Can you work these out from the model? Positions are in its coordinate system, mm. A direction names the side the tool comes from. Round coordinates to 2 decimals unless told otherwise and drop trailing zeros. Write each loop counter-clockwise with the first axis right and the second up, starting at its lowest first coordinate (ties: lowest second). Pieces come first, ordered by that corner, then holes. Notation, with made-up numbers: (-18.5, 49.25) -> (20.5, 49.25) arc R30 ccw to (20.5, 86.25) -> close; hole circle Ø5 at (7.5, 79.25). An arc over 180 degrees is marked (long way). Write item = value, one per line. Start each with the question number.
1) For faces 1 (the face through (3.4, 22.58, -11.66)), 2 (the face through (-4, 26, -23)), 3 (the face through (-12.057, 33.505, -11.339)), which set-ups out of +Z, -Z, +X, -X, +Y, -Y let a thin tool reach every point of the face, with its end or its side?
2) I'm going to push flat-ended pins straight in: pin 1 (9 mm diameter, centred on x = -2.5, z = -9.5, fed in from -Y); pin 2 (5.5 mm diameter, centred on x = -1.5, z = -10.5, fed in from +Y). Where does each tip first touch, or does it pass through?
3) Thinking about a two-plate mould opening in X: for faces 4 (the face through (8.84, 26.73, -11.34)), 5 (the face through (-19.5, 33.47, -11.66)), 6 (the face through (12.612, 26, -11)), 7 (the face through (8, 34.075, -11)), which applies, +X half, -X half, draft (parallel to the pull), parting line (faces both ways), or undercut?
4) Imagine slicing it at A-A, the plane x = 7. Please give me the cut outline in (y, z), then the cut area to 3 significant figures.
5) Imagine slicing it at B-B, the plane y = 21.75. Please give me the cut outline in (x, z).
6) If I drill on line 1 (Y direction, x = 7.5, z = -10.25); line 2 (X direction, y = 31.5, z = -15.75); line 3 (X direction, y = 25.5, z = -16), over which ranges is the centre line in solid material (lowest first)?
7) Imagine slicing it at D-D, the plane x = -7. Please give me the cut outline in (y, z), then the cut area to 3 significant figures.
8) Imagine slicing it at C-C, the plane z = -3.5. Please give me the cut outline in (x, y).
from build123d import *

# Parameters (mm, degrees)
SKETCH_1_W          = 32.677388302
SKETCH_1_H          = 15.432977872
EXTRUDE_1_DEPTH     = 23
SKETCH_2_R          = 1.25
SKETCH_2_W          = 15.458117654
SKETCH_2_H          = 9.017063249
CUT_EXTRUDE_1_DEPTH = 24
FILLET_1_R          = 2
FILLET_2_R          = 2


with BuildPart() as part:
    # 草图1 → 凸台-拉伸1 (new body)
    with BuildSketch(Plane.XY):
        with Locations((-3.726697353, 26.358574689)):
            Rectangle(SKETCH_1_W, SKETCH_1_H)
    extrude(amount=-EXTRUDE_1_DEPTH)

    # 草图2 → 切除-拉伸1 (cut, through all)
    with BuildSketch(Plane.XY):
        with Locations((-15.101697353, 26.358574689)):
            Circle(SKETCH_2_R)
        with Locations((7.648302647, 26.358574689)):
            Circle(SKETCH_2_R)
        with Locations((-3.726697353, 18.642085753)):
            Rectangle(SKETCH_2_W, SKETCH_2_H)
        with Locations((-3.726697353, 34.075063626)):
            Rectangle(SKETCH_2_W, SKETCH_2_H)
    extrude(amount=-CUT_EXTRUDE_1_DEPTH, mode=Mode.SUBTRACT)

    # 圆角1
    fillet_1_edges = [part.edges().sort_by_distance(p)[0] for p in [
        (12.611996798, 18.642085753, -11.5),
        (-20.065391504, 18.642085753, -11.5),
        (-20.065391504, 34.075063625, -11.5),
        (12.611996798, 34.075063625, -11.5),
    ]]
    fillet(fillet_1_edges, radius=FILLET_1_R)

    # 圆角2
    fillet_2_edges = [part.edges().sort_by_distance(p)[0] for p in [
        (-11.45575618, 34.075063625, -11.5),
        (4.002361474, 34.075063625, -11.5),
        (-11.45575618, 29.566532001, -11.5),
        (4.002361474, 29.566532001, -11.5),
        (4.002361474, 18.642085753, -11.5),
        (-11.45575618, 18.642085753, -11.5),
        (4.002361474, 23.150617378, -11.5),
        (-11.45575618, 23.150617378, -11.5),
    ]]
    fillet(fillet_2_edges, radius=FILLET_2_R)


solid = part.part
Reported:
q1.face_1 = +Z, -Z, -Y
q1.face_2 = -Z, +X, -X, +Y, -Y
q1.face_3 = +Z, -Z, +Y
q2.pin_1 = 23.15
q2.pin_2 = 29.57
q3.face_4 = undercut
q3.face_5 = -X half
q3.face_6 = +X half
q3.face_7 = draft
q4.outline = (18.64, -23) -> (25.29, -23) -> (25.29, 0) -> (18.64, 0) -> close; (27.43, -23) -> (34.08, -23) -> (34.08, 0) -> (27.43, 0) -> close
q4.area = 306 mm²
q5.outline = (-20.07, -23) -> (-11.36, -23) -> (-11.36, 0) -> (-20.07, 0) -> close; (3.91, -23) -> (12.61, -23) -> (12.61, 0) -> (3.91, 0) -> close
q6.line_1 = 18.64 to 25.12, 27.6 to 34.08
q6.line_2 = -20.07 to -11.45, 4 to 12.61
q6.line_3 = -20.07 to -16.01, -14.19 to 6.74, 8.56 to 12.61
q7.outline = (23.15, -23) -> (29.57, -23) -> (29.57, 0) -> (23.15, 0) -> close
q7.area = 148 mm²
q8.outline = (-20.07, 20.64) arc R2 ccw to (-18.07, 18.64) -> (-13.46, 18.64) arc R2 ccw to (-11.46, 20.64) -> (-11.46, 21.15) arc R2 cw to (-9.46, 23.15) -> (2, 23.15) arc R2 cw to (4, 21.15) -> (4, 20.64) arc R2 ccw to (6, 18.64) -> (10.61, 18.64) arc R2 ccw to (12.61, 20.64) -> (12.61, 32.08) arc R2 ccw to (10.61, 34.08) -> (6, 34.08) arc R2 ccw to (4, 32.08) -> (4, 31.57) arc R2 cw to (2, 29.57) -> (-9.46, 29.57) arc R2 cw to (-11.46, 31.57) -> (-11.46, 32.08) arc R2 ccw to (-13.46, 34.08) -> (-18.07, 34.08) arc R2 ccw to (-20.07, 32.08) -> close; hole circle Ø2.5 at (-15.1, 26.36); hole circle Ø2.5 at (7.65, 26.36)
